Could you check a few things on this model? Use its own coordinates, in mm. A direction names the side the tool comes from. Give positions to 0.01 mm unless a question says otherwise; leave off trailing zeros. Order: outer loops, then holes, each group sorted by start corner. A loop starts at its lowest first (then second) coordinate and runs counter-clockwise, first axis right, second up. Notation, with made-up numbers: M 85,9.25 L 123,9.25 A24 ccw 123,37.25 Z; hole C 83,66.25 d6. An arc over 180 degrees is marked long. Use a Markdown table: item, result. Add a question column.
```python
from build123d import *

# Parameters (mm, degrees)
SKETCH1_R           = 1.55
BOSS_EXTRUDE1_DEPTH = 3
FILLET1_R           = 3
FILLET3_R           = 3


with BuildPart() as part:
    # Sketch1 → Boss-Extrude1 (new body)
    with BuildSketch(Plane(origin=(0, 0, 0), x_dir=(1, 0, 0), z_dir=(0, 1, 0))):
        with BuildLine():
            Line((2, -7.5), (2, 5.5))
            ThreePointArc((2, 5.5), (4, 10.5), (-1, 12.5))
            Line((-1, 12.5), (-1, -7.5))
            ThreePointArc((-1, -7.5), (-2.5, -9), (-4, -7.5))
            Line((-4, -7.5), (-4, 12.5))
            Line((-4, 12.5), (-12.5, 12.5))
            Line((-12.5, 12.5), (-12.5, -12.5))
            Line((-12.5, -12.5), (2, -12.5))
            Line((2, -12.5), (2, -7.5))
        make_face()
        with Locations(Location((-9.5, 9.5, 0), (0, 0, 270))):
            Circle(SKETCH1_R, mode=Mode.SUBTRACT)
        with Locations(Location((-9.5, -9.5, 0), (0, 0, 270))):
            Circle(SKETCH1_R, mode=Mode.SUBTRACT)
    extrude(amount=-BOSS_EXTRUDE1_DEPTH)

    # Fillet1
    fillet1_edges = [part.edges().sort_by_distance(p)[0] for p in [
        (2, -1.5, 12.5),
    ]]
    fillet(fillet1_edges, radius=FILLET1_R)

    # Fillet3
    fillet3_edges = [part.edges().sort_by_distance(p)[0] for p in [
        (-12.5, -1.5, 12.5),
        (-12.5, -1.5, -12.5),
    ]]
    fillet(fillet3_edges, radius=FILLET3_R)


solid = part.part
```
1) For pin 1 (2.5 mm diameter, centred on x = -9.5, z = 9.5, fed in from -Y); pin 2 (0.9 mm diameter, centred on x = -7.5, y = -1.5, fed in from -Z); pin 3 (1.5 mm diameter, centred on x = -2, y = -0.5, fed in from -Z), each with a flat end and sliding along its axis, tell me the tip position at first contact or that it passes through.
2) Please list where these lines run through material, in increasing order: line 1 (X direction, y = -1.55, z = 9.5); line 2 (X direction, y = -1.9, z = 7); line 3 (X direction, y = -1.35, z = -9.5). Write a range as from..to.
3) Suppose I cut it at C-C on x = -8.25. Please give me the cut outline in (y, z), and give its area (3 significant figures).
4) For faces 1 (the face through (-4, -1, -2)), 2 (the face through (-4.2, 0, -0.3)), 3 (the face through (-7, -1, -12.5)), which set-ups out of +Z, -Z, +X, -X, +Y, -Y let a thin tool reach every point of the face, with its end or its side?
5) Suppose I cut it at A-A on z = 4.5. Please give me the cut outline in (x, y).
6) Suppose I cut it at D-D on z = -9. Please give me the cut outline in (x, y).
7) Suppose I cut it at B-B on y = -2.05. Please give me the cut outline in (x, z), and give its area (3 significant figures).
8) We'd pull the mould along X, two halves only. Please class faces 4 (the face through (-5, -1, 12.5)), 5 (the face through (-11.6, -1.52, 11.64)), 6 (the face through (2, -1, 2)), 7 (the face through (-10.44, -1.48, -10.73)): pulls with the +X half, pulls with the -X half, needs draft (parallel to the pull), parting line crosses it, or undercut.
Values found:
| question | item | result |
|---|---|---|
| 1 | pin 1 | passes through |
| 1 | pin 2 | stops at z = -12.5 |
| 1 | pin 3 | stops at z = 8.33 |
| 2 | line 1 | x = -12.5..-11.05, -7.95..2 |
| 2 | line 2 | x = -12.5..-4, -1..2 |
| 2 | line 3 | x = -12.5..-11.05, -7.95..-4, -1..4.27 |
| 3 | outline | M -3,-12.5 L 0,-12.5 L 0,-10.42 L -3,-10.42 Z; M -3,-8.58 L 0,-8.58 L 0,8.58 L -3,8.58 Z; M -3,10.42 L 0,10.42 L 0,12.5 L -3,12.5 Z |
| 3 | area | 64.0 mm^2 |
| 4 | face 1 | -Z, +Y, -Y |
| 4 | face 2 | +Z, -Z, +X, -X, +Y |
| 4 | face 3 | -Z, -X, +Y, -Y |
| 5 | outline | M -12.5,-3 L -4,-3 L -4,0 L -12.5,0 Z; M -1,-3 L 2,-3 L 2,0 L -1,0 Z |
| 6 | outline | M -12.5,-3 L -10.97,-3 L -10.97,0 L -12.5,0 Z; M -8.03,-3 L -4,-3 L -4,0 L -8.03,0 Z; M -1,-3 L 4.31,-3 L 4.31,0 L -1,0 Z |
| 7 | outline | M -12.5,-9.5 A3 ccw -9.5,-12.5 L -4,-12.5 L -4,7.5 A1.5 cw -1,7.5 L -1,-12.5 A3.81 ccw 2,-5.5 L 2,9.5 A3 ccw -1,12.5 L -9.5,12.5 A3 ccw -12.5,9.5 Z; hole C -9.5,-9.5 d3.1; hole C -9.5,9.5 d3.1 |
| 7 | area | 290 mm^2 |
| 8 | face 4 | needs draft |
| 8 | face 5 | pulls with the -X half |
| 8 | face 6 | pulls with the +X half |
| 8 | face 7 | undercut |
